Verification items for the finished model (mm, model axes). A direction names the side the tool comes from. Coordinates: 2 decimals unless noted, no trailing zeros. Order: outer loops, then holes, each group sorted by start corner. A loop starts at its lowest first (then second) coordinate and runs counter-clockwise, first axis right, second up. Notation, with made-up numbers: (-18.75, 65) - (-14.75, 65) arc R14 ccw to (-14.75, 80) - close; hole circle Ø3 at (-31, -18.5). An arc over 180 degrees is marked (long way). Answer as CSV lines item,"result". Start each with the question number.
1. Material ranges on L1, parallel to Y at x = 32.5, z = 0; L2, parallel to X at y = 5.25, z = -10.5; L3, parallel to Z at x = 27.5, y = 0, recorded low to high. Write a range as [from, to].
2. Go/stop test with flat-tipped pins: pin 1 (4 mm diameter, centred on x = 11.5, y = -3, fed in from -Z); pin 2 (3 mm diameter, centred on x = 5.5, z = 2.5, fed in from +Y); pin 3 (5 mm diameter, centred on x = 27, z = 6.5, fed in from +Y); pin 4 (5 mm diameter, centred on x = 15.5, z = -9, fed in from +Y). Record where each tip stops, or that it passes through.
3. Mould release check, pull along Y, two halves, no side actions. Record for faces 1 (the cylindrical face through (4.93, -0.53, -11.99)), 2 (the cylindrical face through (17.035, -3.186, -1.847)), 3 (the flat face through (0, 0, 0)): pulls with the +Y half, pulls with the -Y half, needs draft (parallel to the pull), parting line crosses it, or undercut.
4. Section check A-A (x = 22.5). Record the cut outline in (y, z).
5. Set-up check for faces 4 (the flat face through (32.7, 0.5, 4.8)), 5 (the cylindrical face through (42.97, 7.42, 4.15)), 6 (the flat face through (32.672, -3.36, -2.517)), 7 (the flat face through (10, -0.2, -5.2)), 8 (the cylindrical face through (43, -0.1, -8.5)): record each of +Z, -Z, +X, -X, +Y, -Y from which the full face is reachable in a straight line by a thin tool's end or side.
from build123d import *

# Parameters (mm, degrees)
F2_SIZE  = 1
F4_DEPTH = 0.5
F5_COUNT = 3


with BuildPart() as f1:
    # F0 (on Front) → F1 (revolve)
    with BuildSketch(Plane.XZ):
        Polygon((40, 5), (10, 5), (10, 12), (0, 12), (0, 0), (8.4978484524, 0), (10, 2.5), (44, 2.5), (44, 5.5), (50, 5.5), (50, 6.5), (45, 8.5), (40, 8.5), align=None)
    revolve(axis=Axis((4.2489242262, 0, 0), (1, 0, 0)))

    # F2
    f2_edges = [f1.edges().sort_by_distance(p)[0] for p in [
        (40, 0, -8.5),
    ]]
    chamfer(f2_edges, length=F2_SIZE)


with BuildPart() as f4:
    # F3 (on Front) → F4 (new body, symmetric)
    with BuildSketch(Plane.XZ):
        with BuildLine():
            Line((56.1913425727, 38), (31, 38))
            ThreePointArc((31, 38), (11, 18), (31, -2))
            Line((31, -2), (56.1913425727, -2))
            Line((56.1913425727, -2), (56.1913425727, 38))
        make_face()
    extrude(amount=F4_DEPTH, both=True)


with BuildPart() as f5_1:
    # F5: instance of F4
    add(f4.part.rotate(Axis((62.4550534707, 0, 0), (1, 0, 0)), 1 * 360 / F5_COUNT))


with BuildPart() as f5_2:
    # F5: instance of F4
    add(f4.part.rotate(Axis((62.4550534707, 0, 0), (1, 0, 0)), 2 * 360 / F5_COUNT))


with BuildPart() as f1_1:
    add(f1.part)

    # F6: cut F4, F5_1, F5_2
    add(f4.part, mode=Mode.SUBTRACT)
    add(f5_1.part, mode=Mode.SUBTRACT)
    add(f5_2.part, mode=Mode.SUBTRACT)


solid = f1_1.part
Evaluation:
1,L1,"y = [-5, -2.5], [2.5, 5]"
1,L2,"x = [0, 10]"
1,L3,"z = [-5, -2.5]"
2,pin 1,"stops at z = -11.88"
2,pin 2,"stops at y = 11.96"
2,pin 3,"stops at y = 3"
2,pin 4,"passes through"
3,face 1,"parting line crosses it"
3,face 2,"undercut"
3,face 3,"needs draft"
4,outline,"(-4.56, -2.05) - (-2.37, -0.79) arc R2.5 cw to (-0.5, 2.45) - (-0.5, 4.97) arc R5 ccw to start; (-4.06, -2.92) arc R5 ccw to (4.06, -2.92) - (1.87, -1.66) arc R2.5 cw to (-1.87, -1.66) - close; (0.5, 2.45) arc R2.5 cw to (2.37, -0.79) - (4.56, -2.05) arc R5 ccw to (0.5, 4.97) - close"
5,face 4,"+Z, +X"
5,face 5,"+X, +Y"
5,face 6,"+X"
5,face 7,"none"
5,face 8,"-Z, +X"
